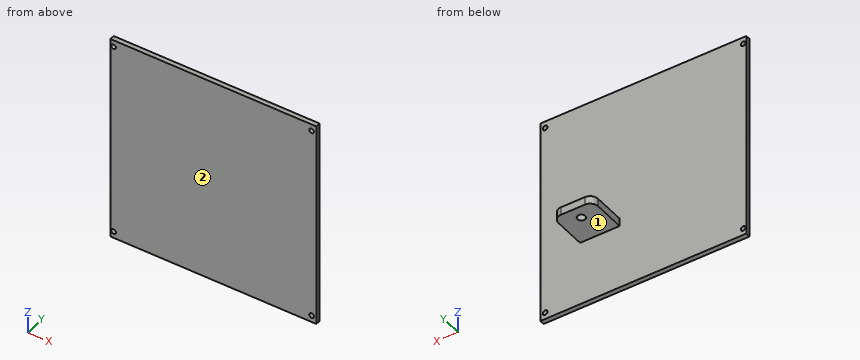
from build123d import *

# Parameters (mm, degrees)
SKETCH1_W           = 130
SKETCH1_H           = 132
BOSS_EXTRUDE1_DEPTH = 3
SKETCH2_W           = 25
SKETCH2_H           = 5
BOSS_EXTRUDE2_DEPTH = 25
FILLET1_R           = 5
SKETCH3_R           = 2.5
CUT_EXTRUDE1_DEPTH  = 25
SKETCH4_R           = 1.5
CUT_EXTRUDE2_DEPTH  = 25


with BuildPart() as part:
    # Sketch1 → Boss-Extrude1 (new body)
    with BuildSketch(Plane(origin=(0, 0, 0), x_dir=(1, 0, 0), z_dir=(0, 1, 0))):
        Rectangle(SKETCH1_W, SKETCH1_H)
    extrude(amount=BOSS_EXTRUDE1_DEPTH)

    # Sketch2 → Boss-Extrude2 (add)
    with BuildSketch(Plane(origin=(0, 3, 0), x_dir=(1, 0, 0), z_dir=(0, 1, 0))):
        with Locations((27.5, 22.5)):
            Rectangle(SKETCH2_W, SKETCH2_H)
    extrude(amount=BOSS_EXTRUDE2_DEPTH)

    # Fillet1
    fillet1_edges = [part.edges().sort_by_distance(p)[0] for p in [
        (15, 28, -22.5),
        (40, 28, -22.5),
    ]]
    fillet(fillet1_edges, radius=FILLET1_R)

    # Sketch3 → Cut-Extrude1 (cut)
    with BuildSketch(Plane.XY.offset(-20)):
        with Locations((27.5, 20.0647296)):
            Circle(SKETCH3_R)
    extrude(amount=-CUT_EXTRUDE1_DEPTH, mode=Mode.SUBTRACT)

    # Sketch4 → Cut-Extrude2 (cut)
    with BuildSketch(Plane(origin=(0, 3, 0), x_dir=(1, 0, 0), z_dir=(0, 1, 0))):
        with Locations(Location((-63, 61.73, 0), (0, 0, 270))):
            Circle(SKETCH4_R)
        with Locations(Location((62, 61.73, 0), (0, 0, 270))):
            Circle(SKETCH4_R)
        with Locations(Location((-63, -61.73, 0), (0, 0, 270))):
            Circle(SKETCH4_R)
        with Locations(Location((62, -61.73, 0), (0, 0, 270))):
            Circle(SKETCH4_R)
    extrude(amount=-CUT_EXTRUDE2_DEPTH, mode=Mode.SUBTRACT)


solid = part.part
Check sheet for the modelled part. Datum: model origin and axes. Units: mm. Face numbers are marked on the shaded views. A direction names the side the tool comes from. Give positions to 0.01 mm unless a question says otherwise; leave off trailing zeros. Loops run counter-clockwise (first coordinate to the right, second up) from the corner with the lowest first, then second, coordinate; pieces in that order, holes last. Notation, with made-up numbers: M 21,51.25 L 43,51.25 A7 ccw 43,56.25 Z; hole C -24,85.25 d5. An arc over 180 degrees is marked long. Use a Markdown table: item, result. Add a question column.
Q1. Go/stop test with flat-tipped pins: pin 1 (5.5 mm diameter, centred on y = 13, z = -23.5, fed in from +X); pin 2 (4 mm diameter, centred on y = 8.5, z = -22, fed in from -X); pin 3 (8 mm diameter, centred on x = 15.5, y = 19.5, fed in from -Z). Record where each tip stops, or that it passes through.
Q2. Sectioned sample at B-B, the plane z = -61.73. Record the cut outline in (x, y).
Q3. Sectioned sample at D-D, the plane y = 15.25. Record the cut outline in (x, z), then the cut area to 3 significant figures.
Q4. Scan lines: line 1 along X through (y, z) = (2.15, 61.73); line 2 along Y through (x, z) = (28, -45.5); line 3 along Z through (x, y) = (23, 23.25). Record each from-to range of solid material in increasing order. Write a range as [from, to].
Q5. Tool access check on the marked faces 1 and 2. Record the directions out of +Z, -Z, +X, -X, +Y, -Y that give a thin tool (end or side, any length) a straight path to the whole face; none if there is none.
Q6. Sectioned sample at A-A, the plane x = -63. Record the cut outline in (y, z), then the cut area to 3 significant figures.
Q7. Sectioned sample at C-C, the plane x = 27.5. Record the cut outline in (y, z).
Verdict:
| question | item | result |
|---|---|---|
| 1 | pin 1 | x = 40 |
| 1 | pin 2 | x = 15 |
| 1 | pin 3 | z = -25 |
| 2 | outline | M -65,0 L -64.5,0 L -64.5,3 L -65,3 Z; M -61.5,0 L 60.5,0 L 60.5,3 L -61.5,3 Z; M 63.5,0 L 65,0 L 65,3 L 63.5,3 Z |
| 3 | outline | M 15,-25 L 40,-25 L 40,-20 L 15,-20 Z |
| 3 | area | 125 mm^2 |
| 4 | line 1 | [-65, -64.5], [-61.5, 60.5], [63.5, 65] |
| 4 | line 2 | [0, 3] |
| 4 | line 3 | [-25, -20] |
| 5 | face 1 | -Z, +X, -X, +Y |
| 5 | face 2 | +Z, -Z, +X, -X, -Y |
| 6 | outline | M 0,-66 L 3,-66 L 3,-63.23 L 0,-63.23 Z; M 0,-60.23 L 3,-60.23 L 3,60.23 L 0,60.23 Z; M 0,63.23 L 3,63.23 L 3,66 L 0,66 Z |
| 6 | area | 378 mm^2 |
| 7 | outline | M 0,-66 L 3,-66 L 3,-25 L 17.56,-25 L 17.56,-20 L 3,-20 L 3,66 L 0,66 Z; M 22.56,-25 L 28,-25 L 28,-20 L 22.56,-20 Z |
